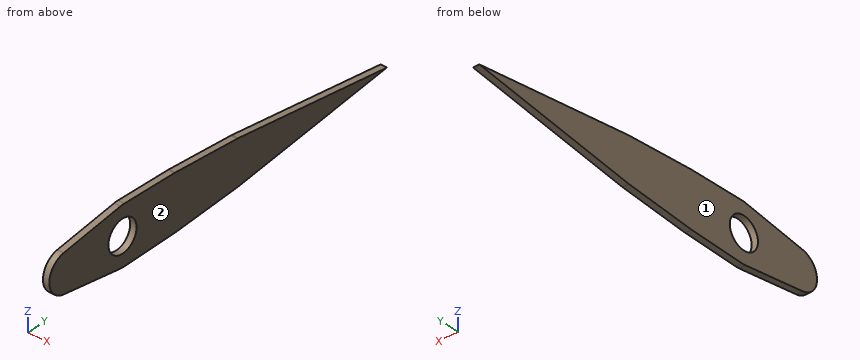
```python
from build123d import *

# Parameters (mm, degrees)
F0_R        = 12.5
F1_DEPTH    = 2.5
F2_T1_DEPTH = 13.4446230753
F2_T3_DEPTH = 7.5224052146
F2_T5_DEPTH = 7.8412582898


# Not quite as in the source:
# - a fillet or chamfer that OpenCascade refuses, or shapes differently, is made with other operations: its cross-section is extruded or revolved along the edge and cut away or added


with BuildPart() as f1:
    # F0 (on Right) → F1 (new body, symmetric)
    with BuildSketch(Plane.YZ):
        with BuildLine():
            Line((102.2685185185, -17.3523434651), (235, 0))
            Line((235, 0), (102.2685185185, 17.3523434651))
            Line((102.2685185185, 17.3523434651), (46.4815775576, 21.4424473282))
            Line((46.4815775576, 21.4424473282), (0, 22.5))
            Line((0, 22.5), (-52.1784368395, 14.8409707545))
            ThreePointArc((-52.1784368395, 14.8409707545), (-65, 0), (-52.1784368395, -14.8409707545))
            Line((-52.1784368395, -14.8409707545), (0, -22.5))
            Line((0, -22.5), (46.4815775576, -21.4424473282))
            Line((46.4815775576, -21.4424473282), (102.2685185185, -17.3523434651))
        make_face()
        Circle(F0_R, mode=Mode.SUBTRACT)
    extrude(amount=F1_DEPTH, both=True)

    # F2: fillet of radius 20 on 4 edges, made by hand

    # F2_s2 → F2_t1 (cut)
    with BuildSketch(Plane.YZ.offset(-6.7223115376)):
        with BuildLine():
            ThreePointArc((-1.6710187212, 22.25471896), (0.0043749886, 22.428949593), (1.6884876427, 22.4615833904))
            Line((1.6884876427, 22.4615833904), (0, 22.5))
            Line((0, 22.5), (-1.6710187212, 22.25471896))
        make_face()
        with BuildLine():
            ThreePointArc((1.6884876427, -22.4615833904), (0.0043749886, -22.428949593), (-1.6710187212, -22.25471896))
            Line((-1.6710187212, -22.25471896), (0, -22.5))
            Line((0, -22.5), (1.6884876427, -22.4615833904))
        make_face()
    extrude(amount=F2_T1_DEPTH, mode=Mode.SUBTRACT)

    # F2_s4 → F2_t3 (cut)
    with BuildSketch(Plane.YZ.offset(-3.7612026073)):
        with BuildLine():
            ThreePointArc((45.9772270381, 21.4539223527), (46.4812725326, 21.4360931288), (46.9847081711, 21.4055595471))
            Line((46.9847081711, 21.4055595471), (46.4815775576, 21.4424473282))
            Line((46.4815775576, 21.4424473282), (45.9772270381, 21.4539223527))
        make_face()
    extrude(amount=F2_T3_DEPTH, mode=Mode.SUBTRACT)

    # F2_s6 → F2_t5 (cut)
    with BuildSketch(Plane.YZ.offset(-3.9206291449)):
        with BuildLine():
            ThreePointArc((101.7017879955, 17.3938941697), (102.267699979, 17.3443139587), (102.8319755439, 17.2786812132))
            Line((102.8319755439, 17.2786812132), (102.2685185185, 17.3523434651))
            Line((102.2685185185, 17.3523434651), (101.7017879955, 17.3938941697))
        make_face()
    extrude(amount=F2_T5_DEPTH, mode=Mode.SUBTRACT)


solid = f1.part
```
Verification items for the finished model (mm, model axes). Face numbers are marked on the shaded views. Coordinates: 2 decimals unless noted, no trailing zeros. Loops run counter-clockwise (first coordinate to the right, second up) from the corner with the lowest first, then second, coordinate; pieces in that order, holes last. Notation, with made-up numbers: (84, -20) - (110, -20) arc R28 cw to (110, 5) - close; hole circle Ø2 at (-17, 48.5). An arc over 180 degrees is marked (long way). Put each result on its own line as item: value.
Item 1: Section check D-D (y = 182.5). Enter the section's corners in (x, z).
Conclusion:
outline: (-2.5, -6.86) - (2.5, -6.86) - (2.5, 6.86) - (-2.5, 6.86) - close
Item 2: Section check C-C (y = 73). Enter the section's corners in (x, z).
Conclusion:
outline: (-2.5, -19.5) - (2.5, -19.5) - (2.5, 19.5) - (-2.5, 19.5) - close
Item 3: Gauge pin test, flat ends, axial feed: pin 1 Ø2 at (x, z) = (-2, 9) entering from -Y; pin 2 Ø1 at (x, y) = (-1.5, 145.5) entering from +Z. Record the tip position at first contact, or that the pin passes through.
Conclusion:
pin 1: stops at y = -62.69
pin 2: stops at z = 11.77
Item 4: Scan lines: line 1 along Z through (x, y) = (0.1, 0); line 2 along Z through (x, y) = (2.15, -7.5); line 3 along Z through (x, y) = (-0.6, 63). Record each from-to range of solid material in increasing order.
Conclusion:
line 1: z = -22.43 to -12.5, 12.5 to 22.43
line 2: z = -21.4 to -10, 10 to 21.4
line 3: z = -20.23 to 20.23
Item 5: Draft check along X on the marked faces 1 and 2. Enter one of: pulls with the +X half, pulls with the -X half, needs draft (parallel to the pull), parting line crosses it, or undercut.
Conclusion:
face 1: pulls with the -X half
face 2: pulls with the +X half
Item 6: Section check B-B (x = -0.9). Enter the section's corners in (y, z).
Conclusion:
outline: (-52.18, -14.84) - (-1.67, -22.25) arc R20 ccw to (1.69, -22.46) - (46.48, -21.44) - (102.27, -17.35) - (235, 0) - (102.83, 17.28) arc R20 ccw to (101.7, 17.39) - (46.98, 21.41) arc R20 ccw to (45.98, 21.45) - (1.69, 22.46) arc R20 ccw to (-1.67, 22.25) - (-52.18, 14.84) arc R15 ccw to start; hole circle Ø25 at (0, 0)
Item 7: Section check A-A (z = 9). Enter the section's corners in (x, y).
Conclusion:
outline: (-2.5, -62) - (2.5, -62) - (2.5, -8.67) - (-2.5, -8.67) - close; (-2.5, 8.67) - (2.5, 8.67) - (2.5, 166.16) - (-2.5, 166.16) - close
